Here's how the part is built. I have some questions about the finished solid (model axes, mm). A direction names the side the tool comes from. Give positions to 0.01 mm unless a question says otherwise; leave off trailing zeros. Write each loop counter-clockwise with the first axis right and the second up, starting at its lowest first coordinate (ties: lowest second). Pieces come first, ordered by that corner, then holes. Notation, with made-up numbers: (-0.75, 3) -> (36.25, 3) arc R25 ccw to (36.25, 24) -> close; hole circle Ø6 at (77.5, -20). An arc over 180 degrees is marked (long way). Answer as CSV lines item,"result". Start each with the question number.
from build123d import *

# Parameters (mm, degrees)
F0_R     = 2.1
F0_R_2   = 4.5
F1_DEPTH = 5
F3_W     = 57.8866787255
F3_H     = 77.1822407842
F4_DEPTH = 5


with BuildPart() as f1:
    # F0 (on Top) → F1 (new body)
    with BuildSketch(Plane.XY):
        Polygon((50, 12.2797499597), (50, 17.2797499597), (-50, 17.2797499597), (-50, 12.2797499597), (-55, 12.2797499597), (-55, -12.2797499597), (-50, -12.2797499597), (-50, -17.2797499597), (50, -17.2797499597), (50, -12.2797499597), (55, -12.2797499597), (55, 12.2797499597), align=None)
        with Locations((-17.5, 0)):
            Circle(F0_R, mode=Mode.SUBTRACT)
        with Locations((17.5, 0)):
            Circle(F0_R, mode=Mode.SUBTRACT)
        with Locations((0, 8)):
            Circle(F0_R_2, mode=Mode.SUBTRACT)
    extrude(amount=F1_DEPTH)

    # F3 (on offset) → F4 (join)
    with BuildSketch(Plane.YZ.offset(55)):
        Rectangle(F3_W, F3_H)
    extrude(amount=-F4_DEPTH)

    # F5: F1 across plane


with BuildPart() as f1_1:
    add(f1.part)
    add(f1.part.mirror(Plane.YZ))


solid = f1_1.part
Item 1: If we section it at B-B (x = 17.5): Please give me the cut outline in (y, z), and give its area (3 significant figures).
Item 2: If I drill on line 1 (X direction, y = -17, z = -11.5); line 2 (Y direction, x = 0, z = 2); line 3 (Z direction, x = -32, y = 1), over which ranges is the centre line in solid material (lowest first)? Write a range as [from, to].
Item 3: If we section it at C-C (z = 14): Please give me the cut outline in (x, y), and give its area (3 significant figures).
Item 4: If we section it at A-A (y = 0): Please give me the cut outline in (x, z), and give its area (3 significant figures).
Item 5: We'd pull the mould along Y, two halves only. Please class faces 4 (the face through (-15.497, 0.631, 2.465)), 5 (the face through (-53, -28.943, -1)), 6 (the face through (-1, 0, 0)): released by +Y, released by -Y, zero draft, split by the parting line, or undercut.
Item 6: For faces 1 (the face through (-1, 0, 5)), 2 (the face through (-1, -17.28, 2)), 3 (the face through (1, 17.28, 2)), which set-ups out of +Z, -Z, +X, -X, +Y, -Y let a thin tool reach every point of the face, with its end or its side?
Item 7: I'm going to push flat-ended pins straight in: pin 1 (17.5 mm diameter, centred on x = -3.5, y = 3.5, fed in from -Z); pin 2 (5.5 mm diameter, centred on x = -17.5, y = 0, fed in from +Z); pin 3 (2.5 mm diameter, centred on x = 17.5, y = 0, fed in from -Z); pin 4 (2.5 mm diameter, centred on x = -1.5, z = 3.5, fed in from +Y). Where does each tip first touch, or does it pass through?
Item 8: If we section it at D-D (y = 8): Please give me the cut outline in (x, z), and give its area (3 significant figures).
Final values:
1,outline,"(-17.28, 0) -> (-2.1, 0) -> (-2.1, 5) -> (-17.28, 5) -> close; (2.1, 0) -> (17.28, 0) -> (17.28, 5) -> (2.1, 5) -> close"
1,area,"152 mm2"
2,line 1,"[-55, -50], [50, 55]"
2,line 2,"[-17.28, 3.5], [12.5, 17.28]"
2,line 3,"[0, 5]"
3,outline,"(-55, -28.94) -> (-50, -28.94) -> (-50, 28.94) -> (-55, 28.94) -> close; (50, -28.94) -> (55, -28.94) -> (55, 28.94) -> (50, 28.94) -> close"
3,area,"579 mm2"
4,outline,"(-55, -38.59) -> (-50, -38.59) -> (-50, 0) -> (-19.6, 0) -> (-19.6, 5) -> (-50, 5) -> (-50, 38.59) -> (-55, 38.59) -> close; (-15.4, 0) -> (15.4, 0) -> (15.4, 5) -> (-15.4, 5) -> close; (19.6, 0) -> (50, 0) -> (50, -38.59) -> (55, -38.59) -> (55, 38.59) -> (50, 38.59) -> (50, 5) -> (19.6, 5) -> close"
4,area,"1,230 mm2"
5,face 4,"undercut"
5,face 5,"released by -Y"
5,face 6,"zero draft"
6,face 1,"+Z, +Y, -Y"
6,face 2,"+Z, -Z, -Y"
6,face 3,"+Z, -Z, +Y"
7,pin 1,"z = 0"
7,pin 2,"z = 5"
7,pin 3,"through"
7,pin 4,"y = 17.28"
8,outline,"(-55, -38.59) -> (-50, -38.59) -> (-50, 0) -> (-4.5, 0) -> (-4.5, 5) -> (-50, 5) -> (-50, 38.59) -> (-55, 38.59) -> close; (4.5, 0) -> (50, 0) -> (50, -38.59) -> (55, -38.59) -> (55, 38.59) -> (50, 38.59) -> (50, 5) -> (4.5, 5) -> close"
8,area,"1,230 mm2"
